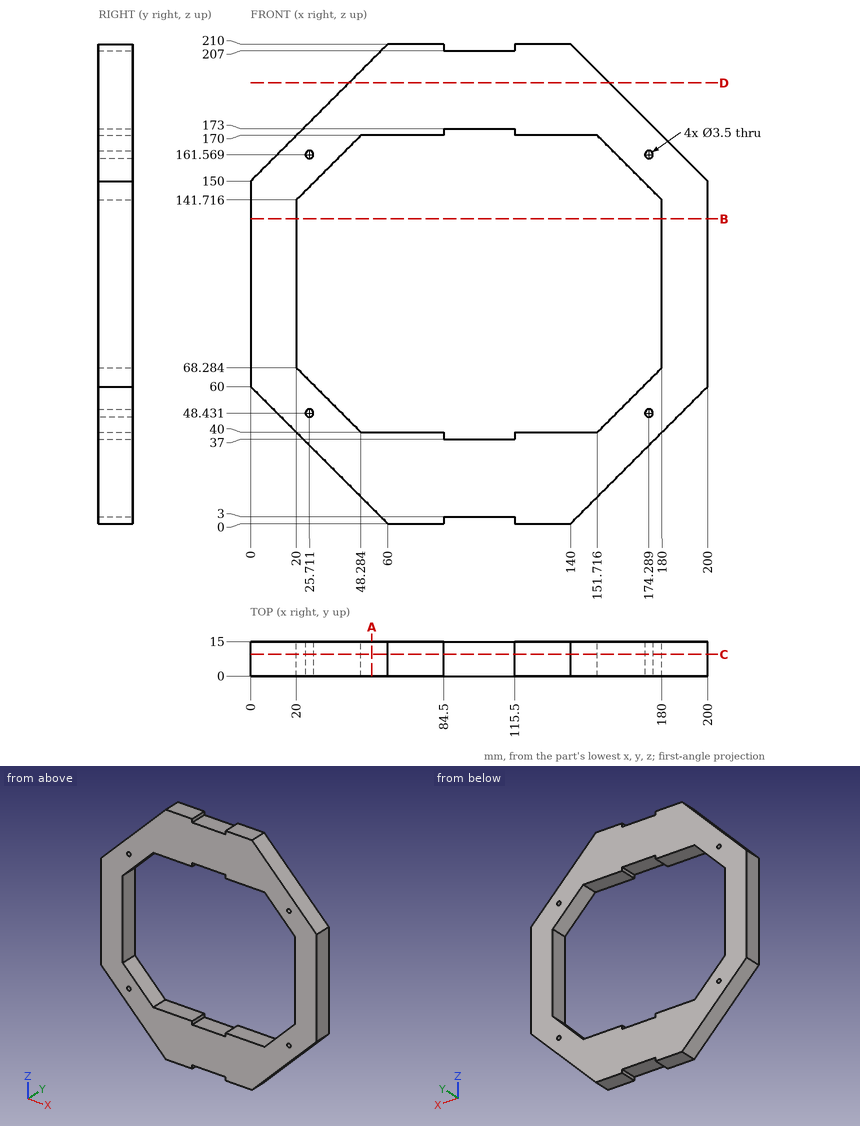
The drawing under review shows one solid part. Ordinate dimensions are in mm from its lowest x, y, z. Coordinates: 2 decimals unless noted, no trailing zeros. Write each loop counter-clockwise with the first axis right and the second up, starting at its lowest first coordinate (ties: lowest second). Pieces come first, ordered by that corner, then holes. Notation, with made-up numbers: (2.5, 61) - (39.5, 61) arc R15 cw to (39.5, 90) - close; hole circle Ø3 at (75.5, 23.5). An arc over 180 degrees is marked (long way). Use one line per item in the form item = value.
Q1. Consider section A-A (x = 53). Write out the cut boundary in (y, z).
Taken from the geometry:
outline = (0, 7) - (15, 7) - (15, 40) - (0, 40) - close; (0, 170) - (15, 170) - (15, 203) - (0, 203) - close
Q2. Consider section B-B (z = 133.5). Write out the cut boundary in (x, y).
Taken from the geometry:
outline = (0, 0) - (20, 0) - (20, 15) - (0, 15) - close; (180, 0) - (200, 0) - (200, 15) - (180, 15) - close
Q3. Insertion check: pin 1 Ø3 at (x, y) = (179.5, 9.5) entering from -Z; pin 2 Ø7.5 at (x, y) = (97, 9) entering from +Z; pin 3 Ø1.5 at (y, z) = (9.5, 209) entering from +X; pin 4 Ø5.5 at (x, z) = (25.71, 48.43) entering from -Y. Each pin has a flat end and moves straight along its axis. Give the tip position at first contact, or say it passes through.
Taken from the geometry:
pin_1 = 38
pin_2 = 207
pin_3 = 141.75
pin_4 = 0
Q4. For probe 1 along X at (y, z) = (10.75, 103.5); probe 2 along Z at (x, y) = (110.5, 12.5); probe 3 along Z at (x, y) = (131, 12.75), list the stretches that pass through material, from the lowest coordinate up.
Taken from the geometry:
probe_1 = 0 to 20, 180 to 200
probe_2 = 3 to 37, 173 to 207
probe_3 = 0 to 40, 170 to 210
Q5. Consider section C-C (y = 9.5). Count the separate pieces of the cut face and the enclosed holes in it, plus the area to 3 significant figures.
Taken from the geometry:
separate_pieces = 1
enclosed_holes = 5
area = 15,200 mm^2
Q6. Consider section D-D (z = 193). Write out the cut boundary in (x, y).
Taken from the geometry:
outline = (43, 0) - (157, 0) - (157, 15) - (43, 15) - close
